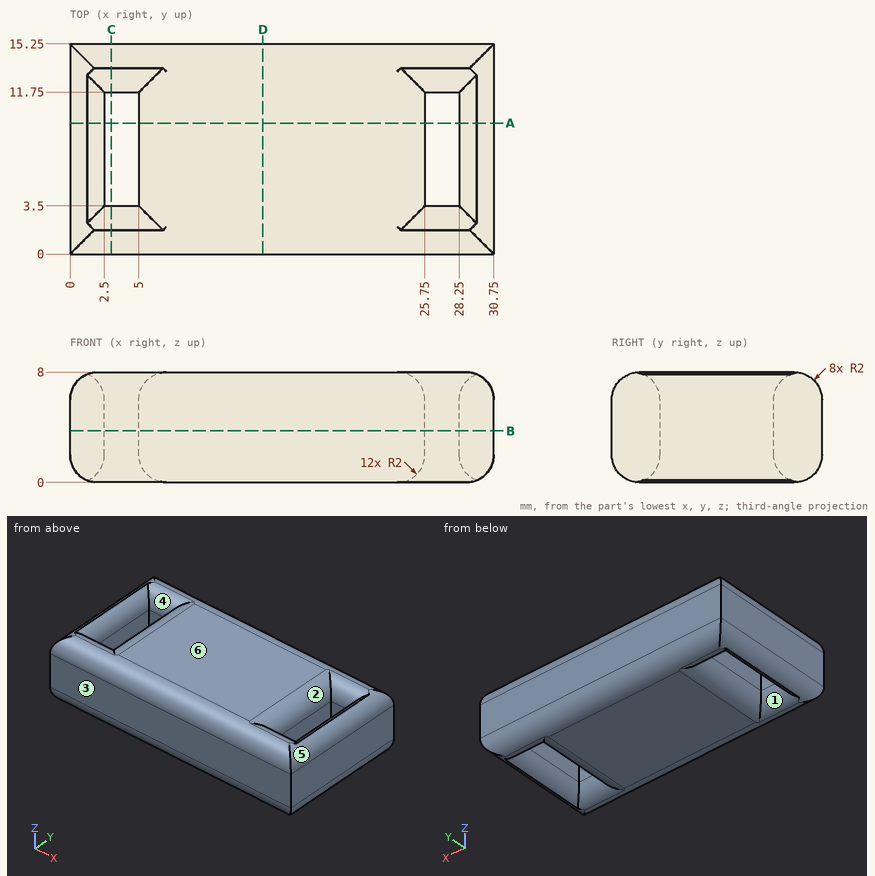
The figure shows three views and two pictorial views of one solid part (mm, origin at its lowest corner). Answer the questions. A direction names the side the tool comes from. Coordinates: 2 decimals unless noted, no trailing zeros. Loops run counter-clockwise (first coordinate to the right, second up) from the corner with the lowest first, then second, coordinate; pieces in that order, holes last. Notation, with made-up numbers: (57, -19.5) - (107, -19.5) arc R20 ccw to (107, 4.5) - close; hole circle Ø8 at (-20, 73). An arc over 180 degrees is marked (long way). Use a Markdown table: item, result. Add a question column.
1) For the marked faces 1, 2 and 3, determine the directions among +Z, -Z, +X, -X, +Y, -Y from which every point of the face is accessible in a straight line to the end or side of a thin tool.
2) Find the intervals of material crossed by line 1 (X direction, y = 8, z = 2.25); line 2 (X direction, y = 9, z = 1); line 3 (Z direction, x = 24.5, y = 12), in increasing order.
3) The part is cut by section C-C, the plane x = 3. Give the vertices of the cut face in (y, z), and give its area (3 significant figures).
4) The part is cut by section B-B, the plane z = 3.75. Give the vertices of the cut face in (x, y), and give its area (3 significant figures).
5) The mould has two halves that part along X. Classify the marked faces 4, 5 and 6: released by +X, released by -X, zero draft, split by the parting line, or undercut.
6) The part is cut by section A-A, the plane y = 9.5. Give the vertices of the cut face in (x, z), and give its area (3 significant figures).
7) The part is cut by section D-D, the plane x = 14. Give the vertices of the cut face in (y, z), and give its area (3 significant figures).
8) Given pin 1 (3 mm diameter, centred on x = 26, y = 10, fed in from -Z), flat-ended and moving along its own axis, determine where the tip first touches the part or whether it passes through.
Here are the results:
| question | item | result |
|---|---|---|
| 1 | face 1 | -Z |
| 1 | face 2 | +Z |
| 1 | face 3 | +Z, -Z, +X, -X, -Y |
| 2 | line 1 | x = 0 to 2.5, 5 to 25.75, 28.25 to 30.75 |
| 2 | line 2 | x = 0.27 to 2.23, 5.27 to 25.48, 28.52 to 30.48 |
| 2 | line 3 | z = 0.15 to 7.85 |
| 3 | outline | (0, 2) arc R2 ccw to (1.75, 0.02) arc R2 ccw to (3.5, 2) - (3.5, 6) arc R2 ccw to (1.75, 7.98) arc R2 ccw to (0, 6) - close; (11.75, 2) arc R2 ccw to (13.5, 0.02) arc R2 ccw to (15.25, 2) - (15.25, 6) arc R2 ccw to (13.5, 7.98) arc R2 ccw to (11.75, 6) - close |
| 3 | area | 49.1 mm^2 |
| 4 | outline | (0, 0) - (30.75, 0) - (30.75, 15.25) - (0, 15.25) - close; hole (2.5, 3.5) - (5, 3.5) - (5, 11.75) - (2.5, 11.75) - close; hole (25.75, 3.5) - (28.25, 3.5) - (28.25, 11.75) - (25.75, 11.75) - close |
| 4 | area | 428 mm^2 |
| 5 | face 4 | undercut |
| 5 | face 5 | released by +X |
| 5 | face 6 | zero draft |
| 6 | outline | (0, 2) arc R2 ccw to (1.25, 0.15) arc R2 ccw to (2.5, 2) - (2.5, 6) arc R2 ccw to (1.25, 7.85) arc R2 ccw to (0, 6) - close; (5, 2) arc R2 ccw to (7, 0) - (23.75, 0) arc R2 ccw to (25.75, 2) - (25.75, 6) arc R2 ccw to (23.75, 8) - (7, 8) arc R2 ccw to (5, 6) - close; (28.25, 2) arc R2 ccw to (29.5, 0.15) arc R2 ccw to (30.75, 2) - (30.75, 6) arc R2 ccw to (29.5, 7.85) arc R2 ccw to (28.25, 6) - close |
| 6 | area | 196 mm^2 |
| 7 | outline | (0, 2) arc R2 ccw to (2, 0) - (13.25, 0) arc R2 ccw to (15.25, 2) - (15.25, 6) arc R2 ccw to (13.25, 8) - (2, 8) arc R2 ccw to (0, 6) - close |
| 7 | area | 119 mm^2 |
| 8 | pin 1 | stops at z = 0.15 |
